```python
from build123d import *

# Parameters (mm, degrees)
Y_KSEKLIK_EKSTR_ZYON1_DEPTH = 2
IZIM2_W                     = 2
IZIM2_H                     = 85.4
Y_KSEKLIK_EKSTR_ZYON2_DEPTH = 2


with BuildPart() as part:
    # Çizim1 → Yükseklik-Ekstrüzyon1 (new body)
    with BuildSketch(Plane.XY):
        with BuildLine():
            Line((-18.3, -48.25), (18.3, -48.25))
            ThreePointArc((18.3, -48.25), (19.714213562, -47.664213562), (20.3, -46.25))
            Line((20.3, -46.25), (20.3, 46.25))
            ThreePointArc((20.3, 46.25), (19.714213562, 47.664213562), (18.3, 48.25))
            Line((18.3, 48.25), (-18.3, 48.25))
            ThreePointArc((-18.3, 48.25), (-19.714213562, 47.664213562), (-20.3, 46.25))
            Line((-20.3, 46.25), (-20.3, -46.25))
            ThreePointArc((-20.3, -46.25), (-19.714213562, -47.664213562), (-18.3, -48.25))
        make_face()
    extrude(amount=Y_KSEKLIK_EKSTR_ZYON1_DEPTH)

    # Çizim2 → Yükseklik-Ekstrüzyon2 (add)
    with BuildSketch(Plane.XY.offset(2)):
        with Locations((-19.3, 0)):
            Rectangle(IZIM2_W, IZIM2_H)
        with Locations((19.3, 0)):
            Rectangle(IZIM2_W, IZIM2_H)
    extrude(amount=Y_KSEKLIK_EKSTR_ZYON2_DEPTH)


solid = part.part
```
Design review of the part built by this model. Coordinates are the model's own, in mm. A direction names the side the tool comes from. Give positions to 0.01 mm unless a question says otherwise; leave off trailing zeros. Order: outer loops, then holes, each group sorted by start corner. A loop starts at its lowest first (then second) coordinate and runs counter-clockwise, first axis right, second up. Notation, with made-up numbers: (-33.5, 12) -> (14.5, 12) arc R14 cw to (14.5, 31) -> close; hole circle Ø11 at (0, -24). An arc over 180 degrees is marked (long way). Write item = value, one per line. Start each with the question number.
(1) For faces 1 (the face through (19, 42.7, 3)), 2 (the face through (20.3, -1, 2)), 3 (the face through (18.3, -1, 3)), 4 (the face through (19, -42.7, 3)), 5 (the face through (19, 1, 4)), list the 3-axis set-ups (+Z, -Z, +X, -X, +Y, -Y) from which the entire face can be reached by the end or side of a thin tool; tool diameter is ignored.
(2) For pin 1 (0.6 mm diameter, centred on x = -19, z = 3.5, fed in from +Y); pin 2 (1.5 mm diameter, centred on x = 6, y = 36.5, fed in from +Z); pin 3 (1 mm diameter, centred on x = 19.5, z = 3, fed in from -Y), all flat-tipped, find the tip position at first contact; note any pin that passes through.
(3) We need section A-A on y = -37.5. Write out the cut boundary in (x, z), plus the area to 3 significant figures.
(4) We need section B-B on x = -7. Write out the cut boundary in (y, z), plus the area to 3 significant figures.
(5) To check wall thickness, follow line 1 along X through (y, z) = (40.5, 3.4); line 2 along Z through (x, y) = (9, 24.5). State the ranges of each line that lie inside material, in increasing order.
Numbers:
q1.face_1 = +Z, +X, -X, +Y
q1.face_2 = +Z, -Z, +X, +Y, -Y
q1.face_3 = +Z, +Y, -Y
q1.face_4 = +Z, +X, -X, -Y
q1.face_5 = +Z, +X, -X, +Y, -Y
q2.pin_1 = 42.7
q2.pin_2 = 2
q2.pin_3 = -42.7
q3.outline = (-20.3, 0) -> (20.3, 0) -> (20.3, 4) -> (18.3, 4) -> (18.3, 2) -> (-18.3, 2) -> (-18.3, 4) -> (-20.3, 4) -> close
q3.area = 89.2 mm^2
q4.outline = (-48.25, 0) -> (48.25, 0) -> (48.25, 2) -> (-48.25, 2) -> close
q4.area = 193 mm^2
q5.line_1 = -20.3 to -18.3, 18.3 to 20.3
q5.line_2 = 0 to 2
